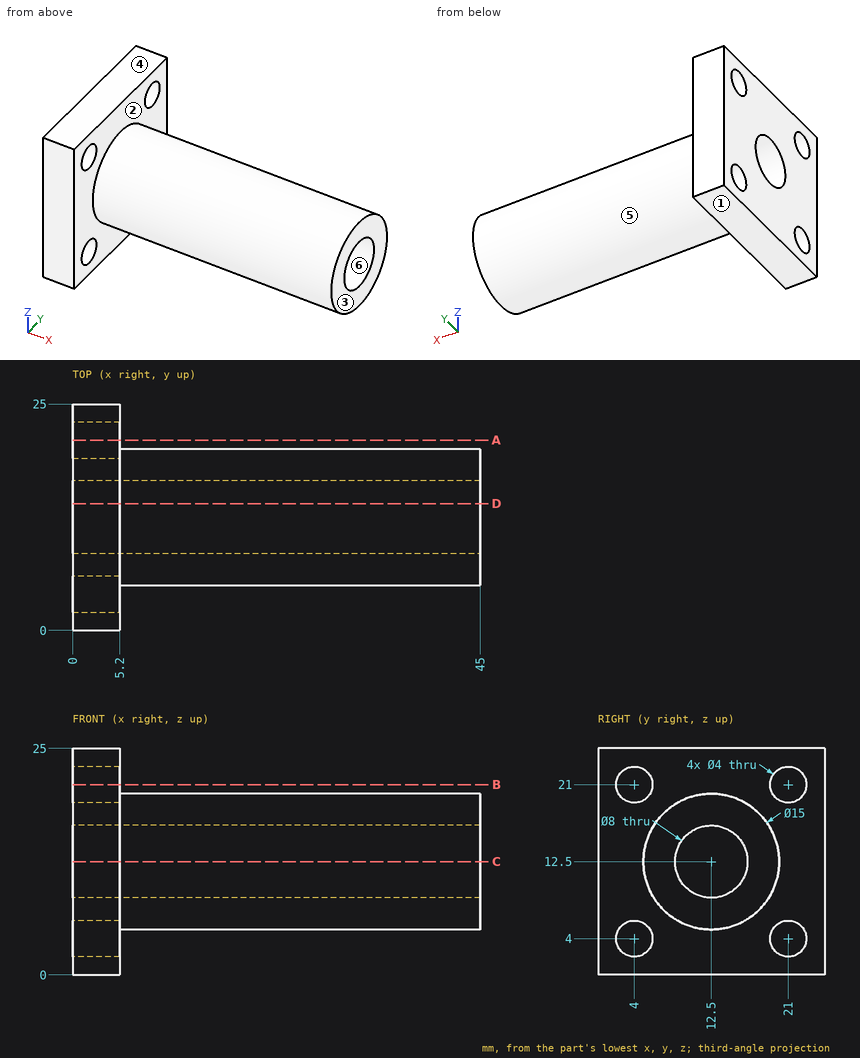
Geometry: see drawing. Coordinates: mm, zero at the bounding-box minimum. A direction names the side the tool comes from. Round coordinates to 2 decimals unless told otherwise and drop trailing zeros. Write each loop counter-clockwise with the first axis right and the second up, starting at its lowest first coordinate (ties: lowest second). Pieces come first, ordered by that corner, then holes. Notation, with made-up numbers: M 50.25,-16.5 L 98.25,-16.5 A3 ccw 98.25,-11.5 Z; hole C -23.5,-40 d8. An arc over 180 degrees is marked long. Answer in a Markdown table with one row per item. Add a question column.
(1) Cut plane A-A, the plane y = 21. Return the cut outline in (x, z).
(2) Draft query along Z for the marked faces 3, 4, 5 and 6. Return one class per face: pulls with the +Z half, pulls with the -Z half, needs draft (parallel to the pull), parting line crosses it, or undercut.
(3) Contact query for flat-ended pins moving along their axis: pin 1 (3 mm diameter, centred on y = 4, z = 4, fed in from +X); pin 2 (10 mm diameter, centred on x = 36, y = 11, fed in from -Z); pin 3 (2 mm diameter, centred on x = 18.5, y = 16.5, fed in from +Z); pin 4 (8 mm diameter, centred on x = 7, y = 5.5, fed in from -Z). Output: stop coordinate, or through.
(4) Cut plane C-C, the plane z = 12.5. Return the cut outline in (x, y).
(5) Reachability of the marked faces 1 and 2 from +Z, -Z, +X, -X, +Y, -Y: full face, straight path, thin tool, end or side. Return the list, or none.
(6) Cut plane D-D, the plane y = 14. Return the cut outline in (x, z).
(7) Ray query, L1, parallel to Z at x = 1.95, y = 21; L2, parallel to Z at x = 25, y = 12.25; L3, parallel to Y at x = 4, z = 20. Return the intervals inside material, ascending.
Established:
| question | item | result |
|---|---|---|
| 1 | outline | M 0,0 L 5.2,0 L 5.2,2 L 0,2 Z; M 0,6 L 5.2,6 L 5.2,19 L 0,19 Z; M 0,23 L 5.2,23 L 5.2,25 L 0,25 Z |
| 2 | face 3 | needs draft |
| 2 | face 4 | pulls with the +Z half |
| 2 | face 5 | parting line crosses it |
| 2 | face 6 | undercut |
| 3 | pin 1 | through |
| 3 | pin 2 | z = 5 |
| 3 | pin 3 | z = 19.37 |
| 3 | pin 4 | z = 0 |
| 4 | outline | M 0,0 L 5.2,0 L 5.2,5 L 45,5 L 45,8.5 L 0,8.5 Z; M 0,16.5 L 45,16.5 L 45,20 L 5.2,20 L 5.2,25 L 0,25 Z |
| 5 | face 1 | -Z, +X, -X, +Y, -Y |
| 5 | face 2 | +X |
| 6 | outline | M 0,0 L 5.2,0 L 5.2,5.15 L 45,5.15 L 45,8.79 L 0,8.79 Z; M 0,16.21 L 45,16.21 L 45,19.85 L 5.2,19.85 L 5.2,25 L 0,25 Z |
| 7 | L1 | 0 to 2, 6 to 19, 23 to 25 |
| 7 | L2 | 5 to 8.51, 16.49 to 20 |
| 7 | L3 | 0 to 2.27, 5.73 to 19.27, 22.73 to 25 |
